```python
from build123d import *

# Parameters (mm, degrees)
BOSS_EXTRUDE1_DEPTH = 2
SKETCH1_3_W         = 42.3
SKETCH1_3_H         = 2
BOSS_EXTRUDE2_DEPTH = 25.4
SKETCH1_4_W         = 8.8
SKETCH1_4_H         = 2
BOSS_EXTRUDE3_DEPTH = 25.3
FILLET13_R          = 3
FILLET14_R          = 3
FILLET15_R          = 3
FILLET16_R          = 3
FILLET18_R          = 3
FILLET19_R          = 3
FILLET20_R          = 3
FILLET21_R          = 3
FILLET24_R          = 2.36
FILLET25_R          = 2.36
FILLET26_R          = 2.2
SKETCH2_R           = 2
CUT_EXTRUDE1_DEPTH  = 10
SKETCH3_R           = 1.5
CUT_EXTRUDE2_DEPTH  = 10
SKETCH4_R           = 1.5
CUT_EXTRUDE3_DEPTH  = 10


with BuildPart() as part:
    # Sketch1 → Boss-Extrude1 (new body)
    with BuildSketch(Plane.XY):
        Polygon((21.15, 16.48), (-21.15, 16.48), (-21.15, 9.72), (-21.15, -9.12), (-18.4, -9.12), (18.4, -9.12), (21.15, -9.12), (21.15, 10.22), align=None)
        with BuildLine():
            Line((-4.349812535, -18.48), (13.96, -18.48))
            ThreePointArc((13.96, -18.48), (17.099554108, -17.179554108), (18.4, -14.04))
            Line((18.4, -14.04), (18.4, -9.12))
            Line((18.4, -9.12), (-18.4, -9.12))
            Line((-18.4, -9.12), (-18.4, -14.04))
            ThreePointArc((-18.4, -14.04), (-17.099554108, -17.179554108), (-13.96, -18.48))
            Line((-13.96, -18.48), (-4.349812535, -18.48))
        make_face()
        Polygon((-21.15, -9.12), (-21.15, 9.72), (-29.95, 9.72), (-29.95, -12.78), (-21.15, -12.78), align=None)
        Polygon((29.95, 10.22), (21.15, 10.22), (21.15, -9.12), (21.15, -12.28), (29.95, -12.28), align=None)
    extrude(amount=BOSS_EXTRUDE1_DEPTH)

    # Sketch1<3> → Boss-Extrude2 (add)
    with BuildSketch(Plane.XY):
        with Locations((0, 17.48)):
            Rectangle(SKETCH1_3_W, SKETCH1_3_H)
    extrude(amount=BOSS_EXTRUDE2_DEPTH)

    # Sketch1<4> → Boss-Extrude3 (add)
    with BuildSketch(Plane.XY):
        with Locations((-25.55, -13.78)):
            Rectangle(SKETCH1_4_W, SKETCH1_4_H)
        with Locations((25.55, -13.28)):
            Rectangle(SKETCH1_4_W, SKETCH1_4_H)
    extrude(amount=BOSS_EXTRUDE3_DEPTH)

    # Fillet13
    fillet13_edges = [part.edges().sort_by_distance(p)[0] for p in [
        (-21.15, -13.78, 25.3),
    ]]
    fillet(fillet13_edges, radius=FILLET13_R)

    # Fillet14
    fillet14_edges = [part.edges().sort_by_distance(p)[0] for p in [
        (-29.95, -13.78, 25.3),
    ]]
    fillet(fillet14_edges, radius=FILLET14_R)

    # Fillet15
    fillet15_edges = [part.edges().sort_by_distance(p)[0] for p in [
        (29.95, -13.28, 25.3),
    ]]
    fillet(fillet15_edges, radius=FILLET15_R)

    # Fillet16
    fillet16_edges = [part.edges().sort_by_distance(p)[0] for p in [
        (21.15, -13.28, 25.3),
    ]]
    fillet(fillet16_edges, radius=FILLET16_R)

    # Fillet18
    fillet18_edges = [part.edges().sort_by_distance(p)[0] for p in [
        (21.15, 17.48, 25.4),
    ]]
    fillet(fillet18_edges, radius=FILLET18_R)

    # Fillet19
    fillet19_edges = [part.edges().sort_by_distance(p)[0] for p in [
        (-21.15, 17.48, 25.4),
    ]]
    fillet(fillet19_edges, radius=FILLET19_R)

    # Fillet20
    fillet20_edges = [part.edges().sort_by_distance(p)[0] for p in [
        (29.95, 10.22, 1),
    ]]
    fillet(fillet20_edges, radius=FILLET20_R)

    # Fillet21
    fillet21_edges = [part.edges().sort_by_distance(p)[0] for p in [
        (-29.95, 9.72, 1),
    ]]
    fillet(fillet21_edges, radius=FILLET21_R)

    # Fillet24
    fillet24_edges = [part.edges().sort_by_distance(p)[0] for p in [
        (-25.55, -14.78, 0),
    ]]
    fillet(fillet24_edges, radius=FILLET24_R)

    # Fillet25
    fillet25_edges = [part.edges().sort_by_distance(p)[0] for p in [
        (25.55, -14.28, 0),
    ]]
    fillet(fillet25_edges, radius=FILLET25_R)

    # Fillet26
    fillet26_edges = [part.edges().sort_by_distance(p)[0] for p in [
        (0, 18.48, 0),
    ]]
    fillet(fillet26_edges, radius=FILLET26_R)

    # Sketch2 → Cut-Extrude1 (cut, symmetric)
    with BuildSketch(Plane.XZ.offset(14.28)):
        with Locations(Location((25.05, 19.14, 0), (0, 0, 180))):
            Circle(SKETCH2_R)
        with Locations(Location((25.05, 9.14, 0), (0, 0, 180))):
            Circle(SKETCH2_R)
        with Locations(Location((-25.15, 19.14, 0), (0, 0, 180))):
            Circle(SKETCH2_R)
        with Locations(Location((-25.15, 9.14, 0), (0, 0, 180))):
            Circle(SKETCH2_R)
    extrude(amount=CUT_EXTRUDE1_DEPTH, both=True, mode=Mode.SUBTRACT)

    # Sketch3 → Cut-Extrude2 (cut)
    with BuildSketch(Plane(origin=(0, 18.48, 0), x_dir=(1, 0, 0), z_dir=(0, 1, 0))):
        with Locations(Location((-9.134575671, -14.14, 0), (0, 0, 270))):
            Circle(SKETCH3_R)
        with Locations(Location((-9.134575671, -7.14, 0), (0, 0, 270))):
            Circle(SKETCH3_R)
        with Locations(Location((-2.134575671, -14.14, 0), (0, 0, 270))):
            Circle(SKETCH3_R)
        with Locations(Location((-9.134575671, -21.14, 0), (0, 0, 270))):
            Circle(SKETCH3_R)
        with Locations(Location((-16.134575671, -14.14, 0), (0, 0, 270))):
            Circle(SKETCH3_R)
        with Locations(Location((9.034575671, -14.14, 0), (0, 0, 270))):
            Circle(SKETCH3_R)
        with Locations(Location((9.034575671, -7.14, 0), (0, 0, 270))):
            Circle(SKETCH3_R)
        with Locations(Location((16.034575671, -14.14, 0), (0, 0, 270))):
            Circle(SKETCH3_R)
        with Locations(Location((9.034575671, -21.14, 0), (0, 0, 270))):
            Circle(SKETCH3_R)
        with Locations(Location((2.034575671, -14.14, 0), (0, 0, 270))):
            Circle(SKETCH3_R)
    extrude(amount=-CUT_EXTRUDE2_DEPTH, mode=Mode.SUBTRACT)

    # Sketch4 → Cut-Extrude3 (cut)
    with BuildSketch(Plane(origin=(0, 0, 0), x_dir=(-1, 0, 0), z_dir=(0, 0, -1))):
        with Locations((-9, -4.52)):
            Circle(SKETCH4_R)
        with Locations((0, 4.48)):
            Circle(SKETCH4_R)
        with Locations((9, -4.52)):
            Circle(SKETCH4_R)
        with Locations((0, -13.52)):
            Circle(SKETCH4_R)
        with Locations((0, -4.52)):
            Circle(SKETCH4_R)
    extrude(amount=-CUT_EXTRUDE3_DEPTH, mode=Mode.SUBTRACT)


solid = part.part
```
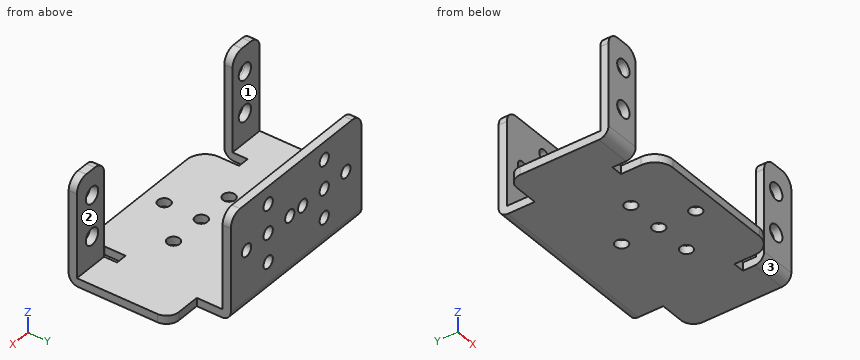
CAD build for the part. Positions are in the model's coordinates, mm. Face numbers are marked on the shaded views. A direction names the side the tool comes from. Round coordinates to 2 decimals unless told otherwise and drop trailing zeros. Write each loop counter-clockwise with the first axis right and the second up, starting at its lowest first coordinate (ties: lowest second). Pieces come first, ordered by that corner, then holes. Notation, with made-up numbers: (47.25, 31) - (79.25, 31) arc R17 ccw to (79.25, 53) - close; hole circle Ø1 at (2.25, -26). An arc over 180 degrees is marked (long way). Return JSON: item names as keys, results as strings. Group by question number.
Item 1: Band-saw the part on D-D on x = 6. List the corners of the cut face in (y, z).
Item 2: Band-saw the part on C-C on y = -4.52. List the corners of the cut face in (x, z).
Item 3: Band-saw the part on A-A on y = 4.48. List the corners of the cut face in (x, z), plus the area to 3 significant figures.
Item 4: Probe probe 1 along X at (y, z) = (17.95, 21.14); probe 2 along X at (y, z) = (-12.9, 9.14); probe 3 along X at (y, z) = (-14, 6.25). List the from-to ranges inside material, lowest first.
Item 5: Band-saw the part on B-B on x = 25.05. List the corners of the cut face in (y, z).
Item 6: 3-axis set-ups, long thin cutter, end or side, ignore diameter. For the marked faces 1, 2 and 3: which of +Z, -Z, +X, -X, +Y, -Y reach the whole face in a straight line?
Item 7: Flat gauge pins, fed straight in: pin 1 Ø2.5 at (x, y) = (0, -13.52) entering from -Z; pin 2 Ø3 at (x, z) = (-4.5, 10) entering from -Y; pin 3 Ø2 at (x, z) = (-22.5, 1) entering from +Y; pin 4 Ø5 at (x, z) = (-25.15, 19.14) entering from -Y. Where does each tip first touch, or does it go through?
Resolved:
{
 "1": {"outline": "(-18.48, 0) - (16.28, 0) arc R2.2 ccw to (18.48, 2.2) - (18.48, 25.4) - (16.48, 25.4) - (16.48, 2) - (-18.48, 2) - close"},
 "2": {"outline": "(-29.95, 0) - (-10.5, 0) - (-10.5, 2) - (-29.95, 2) - close; (-7.5, 0) - (-1.5, 0) - (-1.5, 2) - (-7.5, 2) - close; (1.5, 0) - (7.5, 0) - (7.5, 2) - (1.5, 2) - close; (10.5, 0) - (29.95, 0) - (29.95, 2) - (10.5, 2) - close"},
 "3": {"outline": "(-29.95, 0) - (-1.5, 0) - (-1.5, 2) - (-29.95, 2) - close; (1.5, 0) - (29.95, 0) - (29.95, 2) - (1.5, 2) - close", "area": "114 mm²"},
 "4": {"probe 1": "x = -21.15 to -10.63, -7.63 to 7.53, 10.53 to 21.15", "probe 2": "x = -29.95 to -27.15, -23.15 to -21.15, 21.15 to 23.05, 27.05 to 29.95", "probe 3": "x = -29.95 to -21.15, 21.15 to 29.95"},
 "5": {"outline": "(-14.28, 2.36) arc R2.36 ccw to (-11.92, 0) - (10.22, 0) - (10.22, 2) - (-12.28, 2) - (-12.28, 7.14) - (-14.28, 7.14) - close; (-14.28, 11.14) - (-12.28, 11.14) - (-12.28, 17.14) - (-14.28, 17.14) - close; (-14.28, 21.14) - (-12.28, 21.14) - (-12.28, 25.3) - (-14.28, 25.3) - close"},
 "6": {"face 1": "+Z, -X, +Y", "face 2": "+Z, +X, -X, +Y", "face 3": "-Z, +X, -Y"},
 "7": {"pin 1": "passes through", "pin 2": "stops at y = 16.48", "pin 3": "stops at y = 9.72", "pin 4": "stops at y = -14.78"}
}
